Verification items for the finished model (mm, model axes). Face numbers are marked on the shaded views. A direction names the side the tool comes from. Round coordinates to 2 decimals unless told otherwise and drop trailing zeros. Write each loop counter-clockwise with the first axis right and the second up, starting at its lowest first coordinate (ties: lowest second). Pieces come first, ordered by that corner, then holes. Notation, with made-up numbers: (65, 89.25) -> (95, 89.25) arc R31 cw to (95, 127.25) -> close; hole circle Ø8 at (6.25, 17). An arc over 180 degrees is marked (long way). Answer as a JSON object with one key per item and string values. Group by question number.
(1) Draft check along Y on the marked faces 1, 2 and 3. Enter one of: released by +Y, released by -Y, zero draft, split by the parting line, or undercut.
(2) Scan lines: L1, parallel to Y at x = 0, z = 2.65; L2, parallel to Y at x = -14, z = 4.7; L3, parallel to X at y = -8, z = 0.3. Record each from-to range of solid material in increasing order. Write a range as from..to.
(3) Gauge pin test, flat ends, axial feed: pin 1 Ø1.5 at (x, z) = (-0.5, 0.5) entering from -Y; pin 2 Ø10.5 at (x, y) = (11.79, -11.79) entering from -Z; pin 3 Ø1 at (x, z) = (-16.5, 1) entering from -Y; pin 4 Ø5.5 at (x, y) = (-11.79, 11.79) entering from +Z (3 decimals). Record the tip position at first contact, or that the pin passes through.
(4) Sectioned sample at A-A on x = 0. Record the cut outline in (y, z), and give its area (3 significant figures).
(5) Set-up check for the marked faces 4 and 5: record each of +Z, -Z, +X, -X, +Y, -Y from which the full face is reachable in a straight line by a thin tool's end or side.
(6) Sectioned sample at C-C on z = 0.7. Count the separate pieces of the cut face and the enclosed holes in it, and give its area (3 significant figures).
```python
from build123d import *

# Parameters (mm, degrees)
F0_R            = 24.51608
F0_R_2          = 2.15265
F0_R_3          = 4.7625
F1_DEPTH        = 5.08
F3_DEPTH        = 5.08
F3_COPIES_COUNT = 4
F4_R            = 0.762
F6_R            = 3.96875
F7_DEPTH        = 1.905


# Not quite as in the source:
# - a pattern or mirror of a feature is missing from the dataset's text; its kind, count and spacing are read off the source's solid


with BuildPart() as f1:
    # F0 (on Top) → F1 (new body)
    with BuildSketch(Plane.XY):
        Circle(F0_R)
        with Locations((-11.7865906, -11.7865906)):
            Circle(F0_R_2, mode=Mode.SUBTRACT)
        with Locations((11.7865906, -11.7865906)):
            Circle(F0_R_2, mode=Mode.SUBTRACT)
        with Locations((-11.7865906, 11.7865906)):
            Circle(F0_R_2, mode=Mode.SUBTRACT)
        Circle(F0_R_3, mode=Mode.SUBTRACT)
        with Locations((11.7865906, 11.7865906)):
            Circle(F0_R_2, mode=Mode.SUBTRACT)
    extrude(amount=F1_DEPTH)

    # F2 (on face) → F3 (cut, through all)
    with BuildSketch(Plane.XY.offset(5.08)):
        with BuildLine():
            ThreePointArc((-12.5005198818, 17.2967828873), (-7.4612395718, 15.2741760893), (-6.553034663, 9.9206307084))
            Line((-6.553034663, 9.9206307084), (-3.6703384477, 7.0379344931))
            ThreePointArc((-3.6703384477, 7.0379344931), (0, 7.9375), (3.6703384477, 7.0379344931))
            Line((3.6703384477, 7.0379344931), (6.553034663, 9.9206307084))
            ThreePointArc((6.553034663, 9.9206307084), (7.4612395718, 15.2741760893), (12.5005198818, 17.2967828873))
            ThreePointArc((12.5005198818, 17.2967828873), (0, 21.34108), (-12.5005198818, 17.2967828873))
        make_face()
    f3 = extrude(amount=-F3_DEPTH, mode=Mode.SUBTRACT)

    # F3_copies: F3 ×4 about axis
    f3_copies_axis = Axis((0, 0, 0), (0, 0, 1))
    for i in range(1, F3_COPIES_COUNT):
        add(f3.rotate(f3_copies_axis, i * 360 / F3_COPIES_COUNT), mode=Mode.SUBTRACT)

    # F4
    f4_edges = [f1.edges().sort_by_distance(p)[0] for p in [
        (-12.50052, 17.296783, 2.54),
        (12.50052, 17.296783, 2.54),
        (-17.296783, -12.50052, 2.54),
        (-17.296783, 12.50052, 2.54),
        (12.50052, -17.296783, 2.54),
        (-12.50052, -17.296783, 2.54),
        (17.296783, 12.50052, 2.54),
        (17.296783, -12.50052, 2.54),
    ]]
    fillet(f4_edges, radius=F4_R)

    # F6 (on face) → F7 (cut, through all)
    with BuildSketch(Plane.XY.offset(5.08)):
        with Locations((11.7865906, -11.7865906)):
            Circle(F6_R)
        with Locations((-11.7865906, 11.7865906)):
            Circle(F6_R)
    extrude(amount=-F7_DEPTH, mode=Mode.SUBTRACT)


solid = f1.part
```
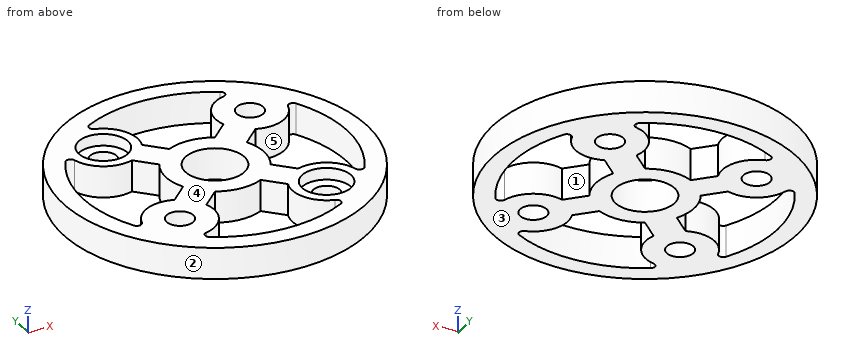
Computed values:
{
 "1": {"face 1": "undercut", "face 2": "split by the parting line", "face 3": "zero draft"},
 "2": {"L1": "-24.52..-21.34, -7.94..-4.76, 4.76..7.94, 21.34..24.52", "L2": "-20.13..-6.69, 6.69..8.49, 15.08..20.13", "L3": "-23.17..-19.78, -15.85..-4.63, 4.63..15.85, 19.78..23.17"},
 "3": {"pin 1": "y = -24.52", "pin 2": "z = 0", "pin 3": "y = -18.58", "pin 4": "z = 3.175"},
 "4": {"outline": "(-24.52, 0) -> (-21.34, 0) -> (-21.34, 5.08) -> (-24.52, 5.08) -> close; (-7.94, 0) -> (-4.76, 0) -> (-4.76, 5.08) -> (-7.94, 5.08) -> close; (4.76, 0) -> (7.94, 0) -> (7.94, 5.08) -> (4.76, 5.08) -> close; (21.34, 0) -> (24.52, 0) -> (24.52, 5.08) -> (21.34, 5.08) -> close", "area": "64.5 mm2"},
 "5": {"face 4": "+Z, +X, -X, +Y, -Y", "face 5": "+Z, -Z"},
 "6": {"separate pieces": "1", "enclosed holes": "9", "area": "971 mm2"}
}
